Geometry check sheet. Reference: the model listing, model coordinates, mm. A direction names the side the tool comes from. Round coordinates to 2 decimals unless told otherwise and drop trailing zeros. Order: outer loops, then holes, each group sorted by start corner. A loop starts at its lowest first (then second) coordinate and runs counter-clockwise, first axis right, second up. Notation, with made-up numbers: (25.25, 44.25) - (56.25, 44.25) arc R26 ccw to (56.25, 62.25) - close; hole circle Ø1 at (-12, 74). An arc over 180 degrees is marked (long way). Return JSON: item names as keys, results as strings. Group by question number.
Q1. Tool access check on faces 4 (the flat face through (-9, 0, 2.5)), 5 (the flat face through (-2, 0, 16)), 6 (the flat face through (-2, 12.5, 3)), 7 (the flat face through (-9, 0, 1.5)), 8 (the flat face through (-1.5, 0, 9)). Record the directions out of +Z, -Z, +X, -X, +Y, -Y that give a thin tool (end or side, any length) a straight path to the whole face; none if there is none.
Q2. Draft check along X on faces 1 (the cylindrical face through (-11.21, 5.45, 1.99)), 2 (the flat face through (-2.5, 0, 9)), 3 (the cylindrical face through (-1.993, -7.67, 8.783)). Enter one of: pulls with the +X half, pulls with the -X half, needs draft (parallel to the pull), parting line crosses it, or undercut.
Q3. Sectioned sample at B-B, the plane y = -7. Record the cut outline in (x, z).
Q4. Gauge pin test, flat ends, axial feed: pin 1 Ø4 at (y, z) = (6, 12.5) entering from +X; pin 2 Ø8 at (x, y) = (-12.5, 7.5) entering from +Z; pin 3 Ø4.5 at (x, y) = (-10.4, -7) entering from -Z. Record the tip position at first contact, or that the pin passes through.
Q5. Sectioned sample at A-A, the plane z = 10.4. Record the cut outline in (x, y).
Q6. Sectioned sample at C-C, the plane x = -10.75. Record the cut outline in (y, z), then the cut area to 3 significant figures.
Q7. Material ranges on line 1 along Y through (x, z) = (-10.4, 1.8); line 2 along X through (y, z) = (5, 12); line 3 along Z through (x, y) = (-10.75, 10.25), recorded low to high.
Q8. Sectioned sample at D-D, the plane y = 10. Record the cut outline in (x, z), then the cut area to 3 significant figures.
```python
from build123d import *

# Parameters (mm, degrees)
EXTRUDE_1_DEPTH     = 12.5
SKETCH_4_R          = 2.121320344
EXTRUDE_3_DEPTH     = 25
SKETCH_5_R          = 1.75
CUT_EXTRUDE_1_DEPTH = 1
SKETCH_6_R          = 1.75
CUT_EXTRUDE_2_DEPTH = 1


with BuildPart() as part:
    # 草图1 → 凸台-拉伸1 (new, symmetric)
    with BuildSketch(Plane(origin=(0, 0, 0), x_dir=(1, 0, 0), z_dir=(0, 1, 0))):
        with BuildLine():
            ThreePointArc((0, -2.5), (1.767766953, 1.767766953), (-2.5, 0))
            Line((-2.5, 0), (-2.5, -1.5))
            Line((-2.5, -1.5), (-16, -1.5))
            Line((-16, -1.5), (-16, -2.5))
            Line((-16, -2.5), (-2.5, -2.5))
            Line((-2.5, -2.5), (-2.5, -16))
            Line((-2.5, -16), (-1.5, -16))
            Line((-1.5, -16), (-1.5, -2.5))
            Line((-1.5, -2.5), (0, -2.5))
        make_face()
        with BuildLine():
            ThreePointArc((-1.5, 0), (1.060660172, 1.060660172), (0, -1.5))
            Line((0, -1.5), (-1.5, -1.5))
            Line((-1.5, -1.5), (-1.5, 0))
        make_face(mode=Mode.SUBTRACT)
    extrude(amount=EXTRUDE_1_DEPTH, both=True)

    # 草图4 → 凸台-拉伸3 (add)
    with BuildSketch(Plane(origin=(0, 12.5, 0), x_dir=(1, 0, 0), z_dir=(0, 1, 0))):
        Circle(SKETCH_4_R)
    extrude(amount=-EXTRUDE_3_DEPTH)

    # 草图5 → 切除-拉伸1 (cut)
    with BuildSketch(Plane(origin=(0, 0, 1.5), x_dir=(-1, 0, 0), z_dir=(0, 0, -1))):
        with Locations((10.4, -7)):
            Circle(SKETCH_5_R)
        with Locations((10.4, 7)):
            Circle(SKETCH_5_R)
    extrude(amount=-CUT_EXTRUDE_1_DEPTH, mode=Mode.SUBTRACT)

    # 草图6 → 切除-拉伸2 (cut)
    with BuildSketch(Plane(origin=(-1.5, 0, 0), x_dir=(0, 0, -1), z_dir=(1, 0, 0))):
        with Locations((-10.4, -7)):
            Circle(SKETCH_6_R)
        with Locations((-10.4, 7)):
            Circle(SKETCH_6_R)
    extrude(amount=-CUT_EXTRUDE_2_DEPTH, mode=Mode.SUBTRACT)


solid = part.part
```
Reply:
{
 "1": {"face 4": "+Z, -X, +Y, -Y", "face 5": "+Z, +X, -X, +Y, -Y", "face 6": "+Z, -Z, +X, -X, +Y", "face 7": "-Z, -X, +Y, -Y", "face 8": "+Z, +X, +Y, -Y"},
 "2": {"face 1": "undercut", "face 2": "pulls with the -X half", "face 3": "needs draft"},
 "3": {"outline": "(-16, 1.5) - (-12.15, 1.5) - (-12.15, 2.5) - (-16, 2.5) - close; (-8.65, 1.5) - (-2.5, 1.5) - (-2.5, 0) arc R2.5 ccw (long way) to (0, 2.5) - (-1.5, 2.5) - (-1.5, 8.65) - (-2.5, 8.65) - (-2.5, 2.5) - (-8.65, 2.5) - close; (-2.5, 12.15) - (-1.5, 12.15) - (-1.5, 16) - (-2.5, 16) - close"},
 "4": {"pin 1": "x = -1.5", "pin 2": "z = 2.5", "pin 3": "z = 1.5"},
 "5": {"outline": "(-2.5, -12.5) - (-1.5, -12.5) - (-1.5, -8.75) - (-2.5, -8.75) - close; (-2.5, -5.25) - (-1.5, -5.25) - (-1.5, 5.25) - (-2.5, 5.25) - close; (-2.5, 8.75) - (-1.5, 8.75) - (-1.5, 12.5) - (-2.5, 12.5) - close"},
 "6": {"outline": "(-12.5, 1.5) - (-8.71, 1.5) - (-8.71, 2.5) - (-12.5, 2.5) - close; (-5.29, 1.5) - (5.29, 1.5) - (5.29, 2.5) - (-5.29, 2.5) - close; (8.71, 1.5) - (12.5, 1.5) - (12.5, 2.5) - (8.71, 2.5) - close", "area": "18.1 mm^2"},
 "7": {"line 1": "-12.5 to -8.75, -5.25 to 5.25, 8.75 to 12.5", "line 2": "-2.5 to -1.5", "line 3": "1.5 to 2.5"},
 "8": {"outline": "(-16, 1.5) - (-2.5, 1.5) - (-2.5, 0) arc R2.5 ccw (long way) to (0, 2.5) - (-1.5, 2.5) - (-1.5, 16) - (-2.5, 16) - (-2.5, 2.5) - (-16, 2.5) - close", "area": "48.0 mm^2"}
}
